Autodesk Inventor part; units mm, degrees
ref_plane "YZ Plane" through (0, 0, 0) normal (1, 0, 0) x (0, 1, 0)
ref_plane "XZ Plane" through (0, 0, 0) normal (0, 1, 0) x (-1, 0, 0)
ref_plane "XY Plane" through (0, 0, 0) normal (0, 0, 1) x (1, 0, 0)
sketch "Sketch1" plane through (0, 0, 0) normal (0, 1, 0) x (-1, 0, 0)
  line L0 (10.5, -9) -> (-10.5, -9)
  line L1 (-10.5, -9) -> (-10.5, 9)
  line L2 (-10.5, 9) -> (10.5, 9)
  line L3 (10.5, 9) -> (10.5, -9)
  point P0 (0, 0)
  point P1 (0, -9)
  point P2 (10.5, 0)
  dimension "d0" = 21
  dimension "d1" = 18
extrude "Extrusion1" add sketch "Sketch1" along normal blind 5
sketch "Sketch2" plane through (-10.5, 0, -9) normal (-1, 0, 0) x (0, 0, 1)
  line L0 (18, 0) -> (10, 0)
  line L1 (10, 0) -> (10, 2)
  line L2 (10, 2) -> (18, 2)
  line L3 (18, 2) -> (18, 0)
  point P0 (9, 0)
  dimension "d4" = 2
  dimension "d5" = 8
extrude "Extrusion2" cut sketch "Sketch2" against normal through all
sketch "Sketch3" plane through (-10.5, 2, 1) normal (0, -1, 0) x (1, 0, 0)
  line L0 (21, 8) -> (21, -10)
  line L1 (21, 0) -> (19.25, 0)
  line L2 (19.25, 0) -> (19.25, 5)
  line L3 (19.25, 5) -> (21, 5)
  line L4 (21, 5) -> (21, 0)
  line L5 (0, -10) -> (0, 8)
  line L6 (0, 0) -> (1.75, 0)
  line L7 (1.75, 0) -> (1.75, 5)
  line L8 (1.75, 5) -> (0, 5)
  line L9 (0, 5) -> (0, 0)
  line L10 (0, 8) -> (21, 8)
  point P0 (10.5, -1)
  point P1 (0, 5)
  dimension "d8" = 5
  dimension "d9" = 3
  dimension "d10" = 17.5
extrude "Extrusion3" cut sketch "Sketch3" against normal through all
sketch "Sketch4" plane through (-10.5, 2, 9) normal (0, -1, 0) x (1, 0, 0)
  line L0 (16.25, -8) -> (4.75, -8)
  line L1 (4.75, -8) -> (4.75, 0)
  line L2 (4.75, 0) -> (16.25, 0)
  line L3 (16.25, 0) -> (16.25, -8)
  line L4 (19.25, -8) -> (19.25, -3)
  line L5 (1.75, -3) -> (1.75, -8)
  point P0 (10.5, -9)
  point P1 (21, 0)
  point P2 (0, -8)
  dimension "d13" = 3
  dimension "d14" = 3
extrude "Extrusion4" cut sketch "Sketch4" against normal through all
chamfer "Chamfer1" distance 2 angle 45 2 edges at (10.5, 3.5, 9) (-10.5, 3.5, 9)
sketch "Sketch6" plane through (10.5, 0, -9) normal (-1, 0, 0) x (0, 0, 1)
  line L0 (10, 5) -> (0, 5)
  line L1 (2.5, 5) -> (5, 5)
  line L2 (5, 5) -> (5, 1)
  line L3 (5, 1) -> (2.5, 1)
  line L4 (2.5, 1) -> (2.5, 5)
  line L5 (0, 0) -> (10, 0)
  line L6 (10, 0) -> (10, 5)
  point P0 (9, 0)
  dimension "d20" = 2.5
  dimension "d22" = 1
  dimension "d23" = 5
chamfer "Chamfer2" distance 2 angle 45 2 edges at (0, 0, 1) (0, 0, -9)
extrude "Extrusion7" cut sketch "Sketch6" along normal blind 12
equation "\"d14\" = d13"
properties part number "Breakout Clip"
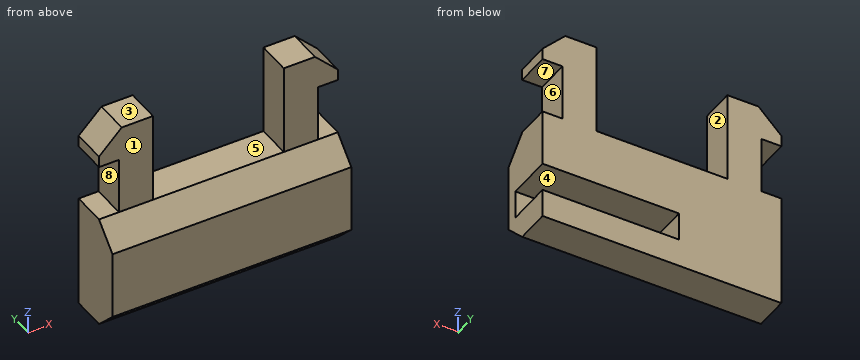
Here's how the part is built. I have some questions about the finished solid (model axes, mm). Face numbers are marked on the shaded views. A direction names the side the tool comes from. Round coordinates to 2 decimals unless told otherwise and drop trailing zeros. Order: outer loops, then holes, each group sorted by start corner. A loop starts at its lowest first (then second) coordinate and runs counter-clockwise, first axis right, second up. Notation, with made-up numbers: (26, -12) -> (78, -12) arc R19 ccw to (78, 16) -> close; hole circle Ø3 at (-19, -19). An arc over 180 degrees is marked (long way). Use CSV: the item, a comma, the result in double quotes.
1. Thinking about a two-plate mould opening in X: for the marked faces 5, 6, 7 and 8, which applies, pulls with the +X half, pulls with the -X half, needs draft (parallel to the pull), parting line crosses it, or undercut?
Recorded:
face 5,"undercut"
face 6,"pulls with the +X half"
face 7,"needs draft"
face 8,"pulls with the -X half"
2. I need wall thicknesses on line 1 along Z through (x, y) = (7.5, 3.4); line 2 along Z through (x, y) = (2.75, 2.5); line 3 along Z through (x, y) = (9.5, 3.8). Which ranges of each line are inside material? Lowest first, please.
Recorded:
line 1,"z = -9 to -6.5, -4 to 9"
line 2,"z = -9 to -6.5, -4 to 1"
line 3,"z = -9 to -6.5, -4 to 1, 6 to 8"
3. Which directions (+Z, -Z, +X, -X, +Y, -Y) give clear straight access to the entire face, cutting with the end or side of a thin tool? Please do the marked faces 1, 2, 3 and 4.
Recorded:
face 1,"+Z, +X, -X, -Y"
face 2,"+Z, +Y, -Y"
face 3,"+Z, +X, -X, +Y, -Y"
face 4,"+X, +Y"
4. I want a section at D-D on z = -5.5. List the corners of the cut face in (x, y) for me, and give its area (3 significant figures).
Recorded:
outline,"(-10.5, 0) -> (10.5, 0) -> (10.5, 1) -> (-1.5, 1) -> (-1.5, 5) -> (-10.5, 5) -> close"
area,"57.0 mm2"
5. I want a section at A-A on z = 3.25. List the corners of the cut face in (x, y) for me, and give its area (3 significant figures).
Recorded:
outline,"(-8.75, 2) -> (-5.75, 2) -> (-5.75, 5) -> (-8.75, 5) -> close; (5.75, 2) -> (8.75, 2) -> (8.75, 5) -> (5.75, 5) -> close"
area,"18.0 mm2"
6. I want a section at B-B on x = 3.25. List the corners of the cut face in (y, z) for me, and give its area (3 significant figures).
Recorded:
outline,"(0, -7) -> (2, -9) -> (5, -9) -> (5, -6.5) -> (1, -6.5) -> (1, -4) -> (5, -4) -> (5, 1) -> (2, 1) -> (0, -1) -> close"
area,"36.0 mm2"
7. I want a section at C-C on y = 2.6. List the corners of the cut face in (x, z) for me.
Recorded:
outline,"(-10.5, -9) -> (10.5, -9) -> (10.5, -6.5) -> (-1.5, -6.5) -> (-1.5, -4) -> (10.5, -4) -> (10.5, 1) -> (8.75, 1) -> (8.75, 6) -> (10.5, 6) -> (10.5, 7) -> (8.5, 9) -> (5.75, 9) -> (5.75, 1) -> (-5.75, 1) -> (-5.75, 9) -> (-8.5, 9) -> (-10.5, 7) -> (-10.5, 6) -> (-8.75, 6) -> (-8.75, 1) -> (-10.5, 1) -> close"
8. I'm going to push flat-ended pins straight in: P1, Ø4, axis at x = -9, z = 7, coming from the -Y side; P2, Ø1.2, axis at x = 5, z = -5.5, coming from the +Y side; P3, Ø3, axis at x = -1, y = 3.5, coming from the +Z side. Where does each tip first touch, or does it pass through?
Recorded:
P1,"stops at y = 2"
P2,"stops at y = 1"
P3,"stops at z = 1"
